from build123d import *

# Parameters (mm, degrees)
F1_DEPTH = 44.45
F2_R     = 5.08


with BuildPart() as f1:
    # F0 (on Right) → F1 (new body, symmetric)
    with BuildSketch(Plane.YZ):
        Polygon((26.359464475, -364.0086964671), (26.359464475, 524.9913035329), (-24.440535525, 524.9913035329), (-24.440535525, 474.1913035329), (-62.540535525, 474.1913035329), (-62.540535525, -275.1086964671), (-24.440535525, -275.1086964671), (-24.440535525, -338.6086964671), (-62.540535525, -338.6086964671), (-62.540535525, -364.0086964671), align=None)
    extrude(amount=F1_DEPTH, both=True)

    # F2
    f2_edges = [f1.edges().sort_by_distance(p)[0] for p in [
        (44.45, -62.540536, 99.541304),
        (44.45, -62.540536, -351.308696),
        (-44.45, -62.540536, -351.308696),
        (-44.45, -62.540536, 99.541304),
        (44.45, 26.359464, 80.491304),
        (-44.45, 26.359464, 80.491304),
    ]]
    fillet(f2_edges, radius=F2_R)


solid = f1.part
Can you work these out from the model? Positions are in its coordinate system, mm. A direction names the side the tool comes from. Give positions to 0.01 mm unless a question says otherwise; leave off trailing zeros. Write each loop counter-clockwise with the first axis right and the second up, starting at its lowest first coordinate (ties: lowest second). Pieces come first, ordered by that corner, then holes. Notation, with made-up numbers: (-11, -16) -> (29, -16) arc R15 cw to (29, -8) -> close; hole circle Ø2 at (34, 4). An arc over 180 degrees is marked (long way). Answer as a JSON object with one key per item and string values. Group by question number.
Item 1: I'm going to push a flat-ended pin straight in: P1, Ø19, axis at x = -7, z = -297.5, coming from the -Y side. Where does the tip first touch, or does it pass through?
Item 2: For faces 5 (the face through (44.45, -19, 87)), 6 (the face through (1, -43, -338.609)), 7 (the face through (1, -43, 474.191)), which set-ups out of +Z, -Z, +X, -X, +Y, -Y let a thin tool reach every point of the face, with its end or its side?
Item 3: Suppose I cut it at B-B (x = -17). Please give me the cut outline in (y, z), plus the area to 3 significant figures.
Item 4: Please list where these lines run through material, in increasing order: line 1 (Z direction, x = -23, y = -29.5); line 2 (Y direction, x = -8, z = -299); line 3 (Y direction, x = -40, z = 431.5). Write a range as [from, to].
Item 5: Suppose I cut it at A-A (y = -45). Please give me the cut outline in (x, z), plus the area to 3 significant figures.
Item 6: We'd pull the mould along Z, two halves only. Please class faces 1 (the face through (1, -44, -275.109)), 2 (the face through (1, 1, 524.991)), 3 (the face through (1, -24.441, -306)), 4 (the face through (-44.45, -19, 87)): +Z half, -Z half, draft (parallel to the pull), parting line (faces both ways), or undercut.
Item 7: Suppose I cut it at C-C (z = -291). Please give me the cut outline in (x, y), plus the area to 3 significant figures.
Findings:
{
 "1": {"P1": "stops at y = -24.44"},
 "2": {"face 5": "+Z, -Z, +X, +Y, -Y", "face 6": "+X, -X, -Y", "face 7": "+Z, +X, -X, -Y"},
 "3": {"outline": "(-62.54, -364.01) -> (26.36, -364.01) -> (26.36, 524.99) -> (-24.44, 524.99) -> (-24.44, 474.19) -> (-62.54, 474.19) -> (-62.54, -275.11) -> (-24.44, -275.11) -> (-24.44, -338.61) -> (-62.54, -338.61) -> close", "area": "74,700 mm²"},
 "4": {"line 1": "z = [-364.01, -338.61], [-275.11, 474.19]", "line 2": "y = [-24.44, 26.36]", "line 3": "y = [-62.5, 26.32]"},
 "5": {"outline": "(-44.45, -364.01) -> (44.45, -364.01) -> (44.45, -338.61) -> (-44.45, -338.61) -> close; (-44.45, -275.11) -> (44.45, -275.11) -> (44.45, 474.19) -> (-44.45, 474.19) -> close", "area": "68,900 mm²"},
 "6": {"face 1": "undercut", "face 2": "+Z half", "face 3": "undercut", "face 4": "draft"},
 "7": {"outline": "(-44.45, -24.44) -> (44.45, -24.44) -> (44.45, 21.28) arc R5.08 ccw to (39.37, 26.36) -> (-39.37, 26.36) arc R5.08 ccw to (-44.45, 21.28) -> close", "area": "4,510 mm²"}
}
